from build123d import *

# Parameters (mm, degrees)
F0_R     = 7.5
F0_R_2   = 1.435
F1_DEPTH = 30
F2_SIZE2 = 0.36397
F2_SIZE  = 1
F4_DEPTH = 10


with BuildPart() as f1:
    # F0 (on Top) → F1 (new body)
    with BuildSketch(Plane.XY):
        Circle(F0_R)
        Circle(F0_R_2, mode=Mode.SUBTRACT)
    extrude(amount=F1_DEPTH)

    # F2
    f2_edges = [f1.edges().sort_by_distance(p)[0] for p in [
        (-1.435, 0, 30),
    ]]
    chamfer(f2_edges, length=F2_SIZE, length2=F2_SIZE2)

    # F3 (on Top) → F4 (join)
    with BuildSketch(Plane.XY):
        with BuildLine():
            ThreePointArc((-3.173077, -6.795703), (-7.5, 0), (-3.173077, 6.795703))
            Line((-3.173077, 6.795703), (-13.846154, 1.812188))
            ThreePointArc((-13.846154, 1.812188), (-15, 0), (-13.846154, -1.812188))
            Line((-13.846154, -1.812188), (-3.173077, -6.795703))
        make_face()
        with BuildLine():
            ThreePointArc((13.846154, -1.812188), (15, 0), (13.846154, 1.812188))
            Line((13.846154, 1.812188), (3.173077, 6.795703))
            ThreePointArc((3.173077, 6.795703), (7.5, 0), (3.173077, -6.795703))
            Line((3.173077, -6.795703), (13.846154, -1.812188))
        make_face()
    extrude(amount=F4_DEPTH)


solid = f1.part
Read the model definition and answer for the solid it produces. Units are mm, in the model's axes. A direction names the side the tool comes from. Coordinates: 2 decimals unless noted, no trailing zeros. Write each loop counter-clockwise with the first axis right and the second up, starting at its lowest first coordinate (ties: lowest second). Pieces come first, ordered by that corner, then holes. Notation, with made-up numbers: M 20,65 L 76,65 A15 cw 76,79 Z; hole C -1,31.5 d3. An arc over 180 degrees is marked long. Use a Markdown table: item, result.
Q1. The part is cut by section C-C, the plane z = 3.75. Write down the section's boundary in (x, y) (3 decimals), then the cut area to 3 significant figures.
Answer block:
| item | result |
|---|---|
| outline | M -13.846,-1.812 L -3.173,-6.796 A7.5 ccw 3.173,-6.796 L 13.846,-1.812 A2 ccw 13.846,1.812 L 3.173,6.796 A7.5 ccw -3.173,6.796 L -13.846,1.812 A2 ccw Z; hole C 0,0 d2.87 |
| area | 276 mm2 |
Q2. The part is cut by section B-B, the plane y = 0. Write down the section's boundary in (x, z) (3 decimals).
Answer block:
| item | result |
|---|---|
| outline | M -15,0 L -1.435,0 L -1.435,29 L -1.799,30 L -7.5,30 L -7.5,10 L -15,10 Z; M 1.435,0 L 15,0 L 15,10 L 7.5,10 L 7.5,30 L 1.799,30 L 1.435,29 Z |
Q3. Determine the mould class of faces 1 (the face through (8.43, -4.34, 4.93)), 2 (the face through (15, 0, 5)), 3 (the face through (0.662, -1.273, 14.297)), 4 (the face through (8.58, 4.27, 4.93)) for opening direction Y: released by +Y, released by -Y, zero draft, split by the parting line, or undercut.
Answer block:
| item | result |
|---|---|
| face 1 | released by -Y |
| face 2 | split by the parting line |
| face 3 | undercut |
| face 4 | released by +Y |
Q4. Which of the six approach directions +Z, -Z, +X, -X, +Y, -Y give full straight-line access (tool end or side, diameter ignored) to faces 5 (the face through (-8.43, 4.34, 4.93)), 6 (the face through (-7.493, 0.33, 18.123))?
Answer block:
| item | result |
|---|---|
| face 5 | +Z, -Z, -X, +Y |
| face 6 | +Z |
Q5. Each of these flat-tipped pins is pushed along its axis until it touches: pin 1 Ø6 at (y, z) = (2.5, 26) entering from -X; pin 2 Ø8 at (x, z) = (-9.5, 26.5) entering from +Y; pin 3 Ø5 at (x, z) = (5.5, 4) entering from +Y. Where does it stop, or does it pass through?
Answer block:
| item | result |
|---|---|
| pin 1 | stops at x = -7.5 |
| pin 2 | stops at y = 5.1 |
| pin 3 | stops at y = 6.87 |
Q6. The part is cut by section D-D, the plane x = 4. Write down the section's boundary in (y, z), then the cut area to 3 significant figures.
Answer block:
| item | result |
|---|---|
| outline | M -6.41,0 L 6.41,0 L 6.41,10 L 6.34,10 L 6.34,30 L -6.34,30 L -6.34,10 L -6.41,10 Z |
| area | 382 mm2 |
Q7. The part is cut by section A-A, the plane x = 0. Write down the section's boundary in (y, z) (3 decimals), then the cut area to 3 significant figures.
Answer block:
| item | result |
|---|---|
| outline | M -7.5,0 L -1.435,0 L -1.435,29 L -1.799,30 L -7.5,30 Z; M 1.435,0 L 7.5,0 L 7.5,30 L 1.799,30 L 1.435,29 Z |
| area | 364 mm2 |
Q8. Straight lines are drawn through the part: L1, parallel to Y at x = 0, z = 6 (3 decimals); L2, parallel to Z at x = -7.5, y = 1.5; L3, parallel to X at y = -0.25, z = 24. For each, find the intervals that lie inside material, in ascending order. Write a range as [from, to].
Answer block:
| item | result |
|---|---|
| L1 | y = [-7.5, -1.435], [1.435, 7.5] |
| L2 | z = [0, 10] |
| L3 | x = [-7.5, -1.41], [1.41, 7.5] |
